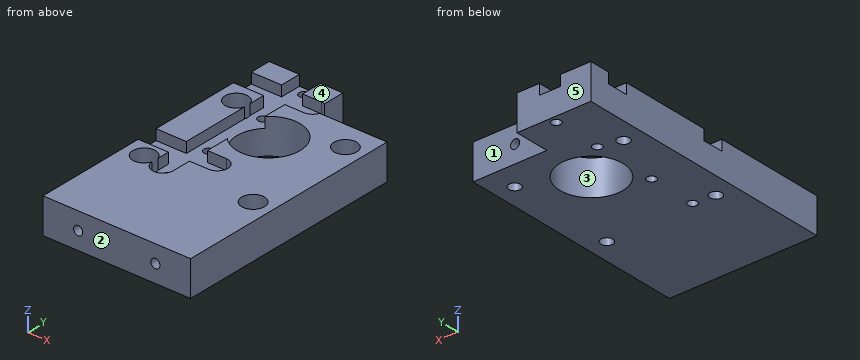
from build123d import *

# Parameters (mm, degrees)
BOSS_EXTRUDE1_DEPTH                      = 10
CUT_EXTRUDE1_REACH                       = 89.407
SKETCH2_R                                = 9
CUT_EXTRUDE2_DEPTH                       = 3
CBORE_FOR_M3_PAN_HEAD_SCREW1_D           = 3.4
CBORE_FOR_M3_PAN_HEAD_SCREW1_CBORE_D     = 6.5
CBORE_FOR_M3_PAN_HEAD_SCREW1_CBORE_DEPTH = 6.5
M3X0_5_TAPPED_HOLE1_D                    = 2.6
M3X0_5_TAPPED_HOLE2_D                    = 2.6
M3X0_5_TAPPED_HOLE2_DEPTH                = 9
M3X0_5_TAPPED_HOLE2_TIP                  = 0.781118805
M3X0_5_TAPPED_HOLE3_D                    = 2.6
M3X0_5_TAPPED_HOLE3_DEPTH                = 9
M3X0_5_TAPPED_HOLE3_TIP                  = 0.781118805


with BuildPart() as part:
    # Sketch1 → Boss-Extrude1 (new body)
    with BuildSketch(Plane.XY):
        Polygon((0, 0), (42, 0), (42, 66), (21, 66), (21, 76), (0, 76), (0, 66), align=None)
    extrude(amount=BOSS_EXTRUDE1_DEPTH)

    # Sketch2 → Cut-Extrude1 (cut, up to next)
    with BuildSketch(Plane.XY.offset(10), mode=Mode.PRIVATE) as cut_extrude1_sk1:
        with Locations((21, 51)):
            Circle(SKETCH2_R)
    cut_extrude1_tool1 = extrude(cut_extrude1_sk1.sketch, amount=-CUT_EXTRUDE1_REACH, mode=Mode.PRIVATE) & part.part
    add(cut_extrude1_tool1.solids().sort_by_distance((21, 51, 10))[0], mode=Mode.SUBTRACT)

    # Sketch3 → Cut-Extrude2 (cut)
    with BuildSketch(Plane.XY.offset(10)):
        with BuildLine():
            Line((8.6, 64), (8.6, 38))
            Line((8.6, 38), (0, 38))
            Line((0, 38), (0, 32))
            Line((0, 32), (8.6, 32))
            Line((8.6, 32), (8.6, 26.6))
            ThreePointArc((8.6, 26.6), (11.6, 23.6), (14.6, 26.6))
            Line((14.6, 26.6), (14.6, 32))
            Line((14.6, 32), (20, 32))
            ThreePointArc((20, 32), (23, 35), (20, 38))
            Line((20, 38), (14.6, 38))
            Line((14.6, 38), (14.6, 64))
            Line((14.6, 64), (20, 64))
            ThreePointArc((20, 64), (23, 67), (20, 70))
            Line((20, 70), (14.6, 70))
            Line((14.6, 70), (14.6, 76))
            Line((14.6, 76), (8.6, 76))
            Line((8.6, 76), (8.6, 70))
            Line((8.6, 70), (0, 70))
            Line((0, 70), (0, 64))
            Line((0, 64), (8.6, 64))
        make_face()
    extrude(amount=-CUT_EXTRUDE2_DEPTH, mode=Mode.SUBTRACT)

    # CBORE for M3 Pan Head Screw1 (through all)
    with Locations(Plane.XY.offset(10)):
        with Locations((5.5, 58.5), (36.5, 58.5), (5.5, 27.5), (36.5, 27.5)):
            CounterBoreHole(CBORE_FOR_M3_PAN_HEAD_SCREW1_D / 2, CBORE_FOR_M3_PAN_HEAD_SCREW1_CBORE_D / 2, CBORE_FOR_M3_PAN_HEAD_SCREW1_CBORE_DEPTH)

    # M3x0.5 Tapped Hole1 (through all)
    with Locations(Plane.XY.offset(7)):
        with Locations((11.6, 73.9), (11.6, 60.1), (11.6, 41.9), (11.6, 28.1)):
            Hole(M3X0_5_TAPPED_HOLE1_D / 2)

    # M3x0.5 Tapped Hole2
    with Locations(Plane(origin=(0, 0, 0), x_dir=(-1, 0, 0), z_dir=(0, -1, 0))):
        with Locations((-32, -5), (-10, -5)):
            Hole(M3X0_5_TAPPED_HOLE2_D / 2, depth=M3X0_5_TAPPED_HOLE2_DEPTH)
            with Locations((0, 0, -(M3X0_5_TAPPED_HOLE2_DEPTH + M3X0_5_TAPPED_HOLE2_TIP / 2))):  # 118° drill point
                Cone(0, M3X0_5_TAPPED_HOLE2_D / 2, M3X0_5_TAPPED_HOLE2_TIP, mode=Mode.SUBTRACT)

    # M3x0.5 Tapped Hole3
    with Locations(Plane(origin=(0, 66, 0), x_dir=(1, 0, 0), z_dir=(0, 1, 0))):
        with Locations((30, -5)):
            Hole(M3X0_5_TAPPED_HOLE3_D / 2, depth=M3X0_5_TAPPED_HOLE3_DEPTH)
            with Locations((0, 0, -(M3X0_5_TAPPED_HOLE3_DEPTH + M3X0_5_TAPPED_HOLE3_TIP / 2))):  # 118° drill point
                Cone(0, M3X0_5_TAPPED_HOLE3_D / 2, M3X0_5_TAPPED_HOLE3_TIP, mode=Mode.SUBTRACT)


solid = part.part
Geometry check sheet. Reference: the model listing, model coordinates, mm. Face numbers are marked on the shaded views. A direction names the side the tool comes from. Round coordinates to 2 decimals unless told otherwise and drop trailing zeros. Write each loop counter-clockwise with the first axis right and the second up, starting at its lowest first coordinate (ties: lowest second). Pieces come first, ordered by that corner, then holes. Notation, with made-up numbers: (21.25, -35.5) - (38.25, -35.5) arc R11 ccw to (38.25, -22.5) - close; hole circle Ø6 at (18.25, 7.25). An arc over 180 degrees is marked (long way). One line per item, written item: value.
1. Scan lines: L1, parallel to Y at x = 36.5, z = 6.5; L2, parallel to Y at x = 5.5, z = 8; L3, parallel to Y at x = 11.6, z = 5.5. Record each from-to range of solid material in increasing order.
The answers:
L1: y = 0 to 24.25, 30.75 to 55.25, 61.75 to 66
L2: y = 0 to 24.25, 30.75 to 32, 38 to 55.25, 61.75 to 64, 70 to 76
L3: y = 0 to 26.8, 29.4 to 40.6, 43.2 to 58.8, 61.4 to 72.6, 75.2 to 76
2. Cross-section at A-A on x = 36.5. Record the boundary of the cut face in (y, z), and give its area (3 significant figures).
The answers:
outline: (0, 0) - (25.8, 0) - (25.8, 3.5) - (24.25, 3.5) - (24.25, 10) - (0, 10) - close; (29.2, 0) - (56.8, 0) - (56.8, 3.5) - (55.25, 3.5) - (55.25, 10) - (30.75, 10) - (30.75, 3.5) - (29.2, 3.5) - close; (60.2, 0) - (66, 0) - (66, 10) - (61.75, 10) - (61.75, 3.5) - (60.2, 3.5) - close
area: 552 mm^2
3. Cross-section at B-B on z = 2. Give the number of separate pieces and of enclosed holes in the cut face, and give its area (3 significant figures).
The answers:
separate pieces: 1
enclosed holes: 9
area: 2,670 mm^2
4. Mould release check, pull along Y, two halves, no side actions. Record for the marked faces 3, 4 and 5: released by +Y, released by -Y, zero draft, split by the parting line, or undercut.
The answers:
face 3: undercut
face 4: zero draft
face 5: released by +Y
5. Cross-section at D-D on y = 33.5. Record the boundary of the cut face in (x, z), and give its area (3 significant figures).
The answers:
outline: (0, 0) - (42, 0) - (42, 10) - (22.6, 10) - (22.6, 7) - (0, 7) - close
area: 352 mm^2
6. Set-up check for the marked faces 1 and 2: record each of +Z, -Z, +X, -X, +Y, -Y from which the full face is reachable in a straight line by a thin tool's end or side.
The answers:
face 1: +Z, -Z, +X, +Y
face 2: +Z, -Z, +X, -X, -Y
7. Cross-section at C-C on x = 16. Record the boundary of the cut face in (y, z), and give its area (3 significant figures).
The answers:
outline: (0, 0) - (43.52, 0) - (43.52, 10) - (38, 10) - (38, 7) - (32, 7) - (32, 10) - (0, 10) - close; (58.48, 0) - (76, 0) - (76, 10) - (70, 10) - (70, 7) - (64, 7) - (64, 10) - (58.48, 10) - close
area: 574 mm^2
8. Depth check by flat-ended pin: pin 1 Ø3.5 at (x, z) = (32, 5) entering from +Y; pin 2 Ø5 at (x, y) = (6, 58.5) entering from +Z. Enter the tip coordinate at first touch or a pass-through.
The answers:
pin 1: stops at y = 66
pin 2: stops at z = 3.5
